from build123d import *

# Parameters (mm, degrees)
F0_W     = 43.610103
F0_H     = 43.610103
F1_DEPTH = 20
F2_R     = 4.915217
F3_DEPTH = 18.3


with BuildPart() as f1:
    # F0 (on Top) → F1 (new body)
    with BuildSketch(Plane.XY):
        with Locations((-21.805051, 21.805051)):
            Rectangle(F0_W, F0_H)
    extrude(amount=F1_DEPTH)

    # F2 (on Right) → F3 (join)
    with BuildSketch(Plane.YZ):
        with Locations((20.946585, 9.500364)):
            Circle(F2_R)
    extrude(amount=F3_DEPTH)


solid = f1.part
Build history of the part. All positions in model axes, mm. A direction names the side the tool comes from. Round coordinates to 2 decimals unless told otherwise and drop trailing zeros. Write each loop counter-clockwise with the first axis right and the second up, starting at its lowest first coordinate (ties: lowest second). Pieces come first, ordered by that corner, then holes. Notation, with made-up numbers: M -40,56 L 15,56 A18 cw 15,86 Z; hole C 30.25,17 d1. An arc over 180 degrees is marked long. Use CSV: the item, a comma, the result in double quotes.
1. Flat gauge pins, fed straight in: pin 1 (12 mm diameter, centred on y = 32.5, z = 16.5, fed in from +X); pin 2 (1.5 mm diameter, centred on x = 11.5, z = 5, fed in from +Y). Where does each tip first touch, or does it go through?
Reply:
pin 1,"stops at x = 0"
pin 2,"stops at y = 24.12"
2. Saw through at C-C (x = 12.5). Give the cut face in (y, z), plus the area to 3 significant figures.
Reply:
outline,"C 20.95,9.5 d9.83"
area,"75.9 mm²"
3. Saw through at B-B (y = 20). Give the cut face in (x, z), plus the area to 3 significant figures.
Reply:
outline,"M -43.61,0 L 0,0 L 0,4.68 L 18.3,4.68 L 18.3,14.32 L 0,14.32 L 0,20 L -43.61,20 Z"
area,"1,050 mm²"
4. Wall check: probe 1 along X at (y, z) = (7, 1.5); probe 2 along Z at (x, y) = (13, 21); probe 3 along Y at (x, z) = (12, 14). Give the ranges that are in metal, low to high. Write a range as from..to.
Reply:
probe 1,"x = -43.61..0"
probe 2,"z = 4.59..14.42"
probe 3,"y = 18.97..22.92"
5. Tool access for faces 1 (the face through (9.022, 19.881, 4.702)), 2 (the face through (-22, 22, 0)): list every direction of +Z, -Z, +X, -X, +Y, -Y with a clear straight run to the whole face (end or side of a thin tool).
Reply:
face 1,"+X"
face 2,"-Z, +X, -X, +Y, -Y"
6. Saw through at A-A (z = 11.5). Give the cut face in (x, y), plus the area to 3 significant figures.
Reply:
outline,"M -43.61,0 L 0,0 L 0,16.46 L 18.3,16.46 L 18.3,25.44 L 0,25.44 L 0,43.61 L -43.61,43.61 Z"
area,"2,070 mm²"
7. Saw through at D-D (y = 38). Give the cut face in (x, z).
Reply:
outline,"M -43.61,0 L 0,0 L 0,20 L -43.61,20 Z"
